from build123d import *

# Parameters (mm, degrees)
F0_W     = 60
F0_H     = 98
F0_W_2   = 50
F0_H_2   = 80
F0_W_3   = 12.190704
F0_H_3   = 3
F1_DEPTH = 1
F3_DEPTH = 3
F4_W     = 57
F4_H     = 96.5
F4_W_2   = 50
F4_H_2   = 80
F4_W_3   = 12.190704
F4_H_3   = 3
F5_DEPTH = 1


with BuildPart() as f1:
    # F0 (on Top) → F1 (new body)
    with BuildSketch(Plane.XY):
        with Locations((0, 6.455527)):
            Rectangle(F0_W, F0_H)
        with Locations((0, 2.455527)):
            Rectangle(F0_W_2, F0_H_2, mode=Mode.SUBTRACT)
        with Locations((0, 48.955527)):
            Rectangle(F0_W_3, F0_H_3, mode=Mode.SUBTRACT)
    extrude(amount=F1_DEPTH)

    # F2 (on face) → F3 (join)
    with BuildSketch(Plane.XY.offset(1)):
        Polygon((-28.5, 55.455527), (-30, 55.455527), (-30, -42.544473), (30, -42.544473), (30, 55.455527), (28.5, 55.455527), (28.5, -41.044473), (-28.5, -41.044473), align=None)
    extrude(amount=F3_DEPTH)

    # F4 (on face) → F5 (join)
    with BuildSketch(Plane.XY.offset(4)):
        with Locations((0, 7.205527)):
            Rectangle(F4_W, F4_H)
        with Locations((0, 2.455527)):
            Rectangle(F4_W_2, F4_H_2, mode=Mode.SUBTRACT)
        with Locations((0, 48.955527)):
            Rectangle(F4_W_3, F4_H_3, mode=Mode.SUBTRACT)
        Polygon((30, -42.544473), (30, 55.455527), (28.5, 55.455527), (28.5, -41.044473), (-28.5, -41.044473), (-28.5, 55.455527), (-30, 55.455527), (-30, -42.544473), align=None)
    extrude(amount=F5_DEPTH)


solid = f1.part
Design review of the part built by this model. Coordinates are the model's own, in mm. A direction names the side the tool comes from. Coordinates: 2 decimals unless noted, no trailing zeros. Order: outer loops, then holes, each group sorted by start corner. A loop starts at its lowest first (then second) coordinate and runs counter-clockwise, first axis right, second up. Notation, with made-up numbers: (-22.5, 4) -> (31.5, 4) arc R21 cw to (31.5, 20) -> close; hole circle Ø4 at (-21, 27). An arc over 180 degrees is marked (long way). Use one line per item in the form item = value. Start each with the question number.
(1) Add section B-B on x = -3. State the section outline as (y, z) points, plus the area to 3 significant figures.
(2) The part is to be moulded in two halves that separate along X. For faces 3 (the flat face through (0, -42.544, 2)), 4 (the flat face through (-2, 43, 1)), 5 (the flat face through (30, 6, 2)), say which applies: +X half, -X half, draft (parallel to the pull), parting line (faces both ways), or undercut.
(3) For probe 1 along Y at (x, z) = (0.5, 0.75); probe 2 along X at (y, z) = (-22.5, 4.5); probe 3 along Y at (x, z) = (16.5, 4.75), list the stretches that pass through material, from the lowest coordinate up.
(4) For faces 1 (the flat face through (-2, 43, 0)), 2 (the flat face through (0, -41.044, 2)), list the 3-axis set-ups (+Z, -Z, +X, -X, +Y, -Y) from which the entire face can be reached by the end or side of a thin tool; tool diameter is ignored.
(5) Add section D-D on x = -13. State the section outline as (y, z) points.
(6) Add section A-A on y = -20. State the section outline as (x, z) points.
(7) Insertion check: pin 1 (1 mm diameter, centred on x = 7, y = 42, fed in from -Z); pin 2 (8 mm diameter, centred on x = -19, y = -30, fed in from +Z). Each pin has a flat end and moves straight along its axis. Give the tip position at first contact, or say it passes through.
(8) Add section C-C on y = 44. State the section outline as (x, z) points, plus the area to 3 significant figures.
Answer block:
q1.outline = (-42.54, 0) -> (-37.54, 0) -> (-37.54, 1) -> (-41.04, 1) -> (-41.04, 4) -> (-37.54, 4) -> (-37.54, 5) -> (-42.54, 5) -> close; (42.46, 0) -> (47.46, 0) -> (47.46, 1) -> (42.46, 1) -> close; (42.46, 4) -> (47.46, 4) -> (47.46, 5) -> (42.46, 5) -> close; (50.46, 0) -> (55.46, 0) -> (55.46, 1) -> (50.46, 1) -> close; (50.46, 4) -> (55.46, 4) -> (55.46, 5) -> (50.46, 5) -> close
q1.area = 34.5 mm²
q2.face_3 = draft
q2.face_4 = undercut
q2.face_5 = +X half
q3.probe_1 = -42.54 to -37.54, 42.46 to 47.46, 50.46 to 55.46
q3.probe_2 = -30 to -25, 25 to 30
q3.probe_3 = -42.54 to -37.54, 42.46 to 55.46
q4.face_1 = -Z, +X, -X, +Y, -Y
q4.face_2 = +Y
q5.outline = (-42.54, 0) -> (-37.54, 0) -> (-37.54, 1) -> (-41.04, 1) -> (-41.04, 4) -> (-37.54, 4) -> (-37.54, 5) -> (-42.54, 5) -> close; (42.46, 0) -> (55.46, 0) -> (55.46, 1) -> (42.46, 1) -> close; (42.46, 4) -> (55.46, 4) -> (55.46, 5) -> (42.46, 5) -> close
q6.outline = (-30, 0) -> (-25, 0) -> (-25, 1) -> (-28.5, 1) -> (-28.5, 4) -> (-25, 4) -> (-25, 5) -> (-30, 5) -> close; (25, 0) -> (30, 0) -> (30, 5) -> (25, 5) -> (25, 4) -> (28.5, 4) -> (28.5, 1) -> (25, 1) -> close
q7.pin_1 = 0
q7.pin_2 = through
q8.outline = (-30, 0) -> (30, 0) -> (30, 5) -> (-30, 5) -> close; hole (-28.5, 1) -> (28.5, 1) -> (28.5, 4) -> (-28.5, 4) -> close
q8.area = 129 mm²
